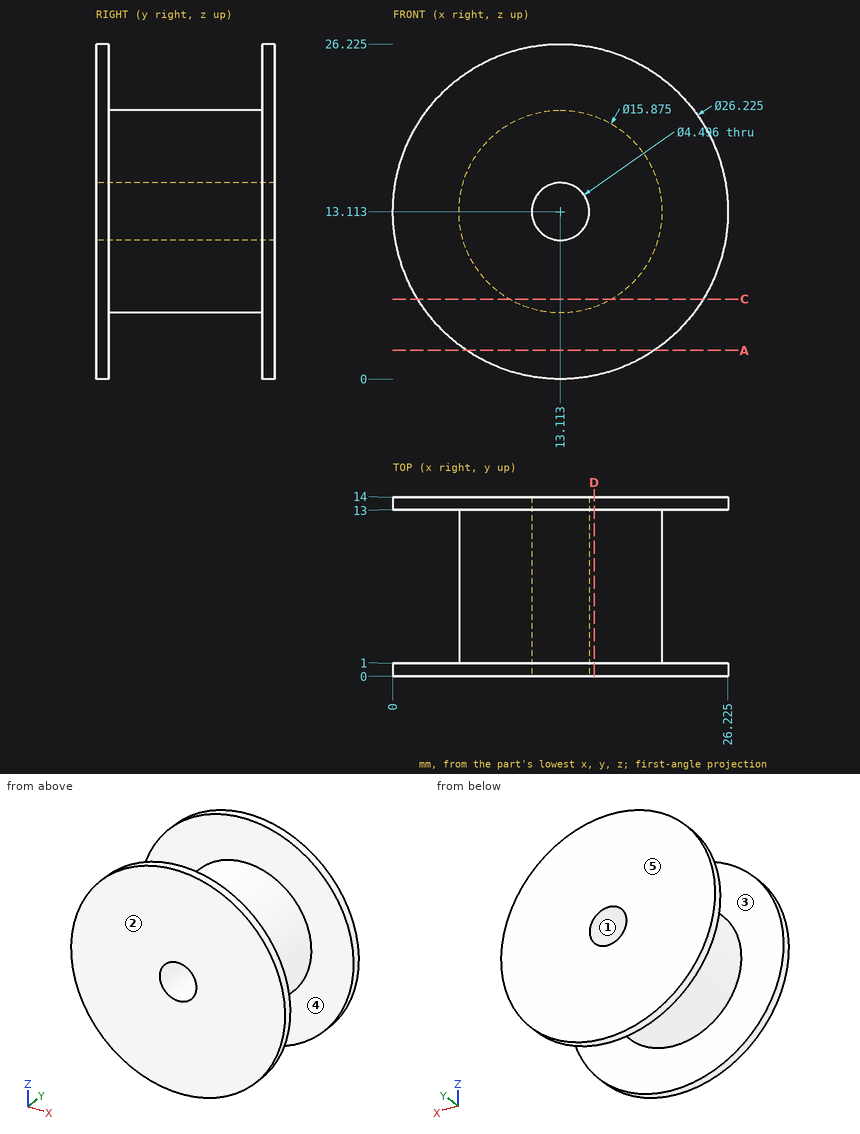
Geometry check sheet. Reference: drawing and pictorial views, mm from the part's lowest x, y, z. A direction names the side the tool comes from. Round coordinates to 2 decimals unless told otherwise and drop trailing zeros. Order: outer loops, then holes, each group sorted by start corner. A loop starts at its lowest first (then second) coordinate and runs counter-clockwise, first axis right, second up. Notation, with made-up numbers: M -38,-27 L -17,-27 A21 cw -17,-10 Z; hole C -18.75,76 d10. An arc over 180 degrees is marked long. One line per item, written item: value. Start each with the question number.
1. Section check C-C on z = 6.25. Enter the section's corners in (x, y) (1 decimal).
2. Release check for a two-part mould opening along Y. For the marked faces 1, 2 and 3 record: released by +Y, released by -Y, zero draft, split by the parting line, or undercut.
3. Section check A-A on z = 2.25. Enter the section's corners in (x, y).
4. Section check D-D on x = 15.75. Enter the section's corners in (y, z), and give its area (3 significant figures).
5. Access from +Z, -Z, +X, -X, +Y, -Y to the whole of each face (thin tool, end or side, straight path). Record for the marked faces 4 and 5.
6. Gauge pin test, flat ends, axial feed: P1, Ø4, axis at x = 13.11, z = 13.11, coming from the +Y side; P2, Ø1.5, axis at y = 9.5, z = 20, coming from the +X side (1 decimal). Record the tip position at first contact, or that the pin passes through.
7. Scan lines: line 1 along Y through (x, z) = (5, 4.25); line 2 along X through (y, z) = (1.75, 13.5) (1 decimal); line 3 along X through (y, z) = (6, 12.25) (1 decimal). Record each from-to range of solid material in increasing order.
Results found:
1. outline: M 1.9,0 L 24.3,0 L 24.3,1 L 17.1,1 L 17.1,13 L 24.3,13 L 24.3,14 L 1.9,14 L 1.9,13 L 9.1,13 L 9.1,1 L 1.9,1 Z
2. face 1: zero draft
2. face 2: released by -Y
2. face 3: undercut
3. outline: M 5.77,0 L 20.46,0 L 20.46,1 L 5.77,1 Z; M 5.77,13 L 20.46,13 L 20.46,14 L 5.77,14 Z
4. outline: M 0,0.27 L 1,0.27 L 1,5.63 L 13,5.63 L 13,0.27 L 14,0.27 L 14,25.96 L 13,25.96 L 13,20.6 L 1,20.6 L 1,25.96 L 0,25.96 Z
4. area: 231 mm^2
5. face 4: none
5. face 5: +Z, -Z, +X, -X, +Y
6. P1: through
6. P2: x = 18.1
7. line 1: 0 to 1, 13 to 14
7. line 2: 5.2 to 10.9, 15.3 to 21
7. line 3: 5.2 to 11, 15.2 to 21
